Verification items for the finished model (mm, model axes). A direction names the side the tool comes from. Coordinates: 2 decimals unless noted, no trailing zeros. Order: outer loops, then holes, each group sorted by start corner. A loop starts at its lowest first (then second) coordinate and runs counter-clockwise, first axis right, second up. Notation, with made-up numbers: (-29.5, -37) -> (-7.5, -37) arc R15 ccw to (-7.5, -22) -> close; hole circle Ø6 at (19, 15). An arc over 180 degrees is marked (long way). Write item = value, one per line. Start each with the question number.
1. Thickness scan on line 1 along X through (y, z) = (31.75, 1.15); line 2 along X through (y, z) = (8.5, 1.55); line 3 along X through (y, z) = (-6, 0.5). Record the ranges inside material, lowest first. Write a range as from..to.
2. Cross-section at C-C on y = 31.75. Record the cut outline in (x, z), plus the area to 3 significant figures.
3. Cross-section at A-A on y = -24.95. Record the cut outline in (x, z), plus the area to 3 significant figures.
4. Set-up check for faces 1 (the flat face through (-5, 3.468, 1)), 2 (the flat face through (-4, 0, -1)), 3 (the cylindrical face through (-4.474, -28.776, 2.986)): record each of +Z, -Z, +X, -X, +Y, -Y from which the full face is reachable in a straight line by a thin tool's end or side.
5. Release check for a two-part mould opening along Y. For faces 4 (the flat face through (-5, -8.005, 1)), 5 (the cylindrical face through (14.73, 34.58, 3.4)), 6 (the cylindrical face through (-40.688, 0.464, 3.399)), 7 (the cylindrical face through (27.8, -25, 1.5)) record: +Y half, -Y half, draft (parallel to the pull), parting line (faces both ways), or undercut.
6. Cross-section at B-B on x = -19.5. Give the number of separate pieces and of enclosed holes in the cut face, plus the area to 3 significant figures.
7. Go/stop test with flat-tipped pins: P1, Ø1, axis at y = 16.5, z = 1.5, coming from the +X side; P2, Ø5, axis at x = -24, y = 19.5, coming from the -Z side; P3, Ø0.5, axis at y = 29.5, z = -0.5, coming from the +X side. Record where each tip stops, or that it passes through.
from build123d import *

# Parameters (mm, degrees)
SKETCH141_W          = 73.258
SKETCH141_H          = 70.3
SKETCH141_R          = 1.75
PAD050_DEPTH         = 4
FILLET012_R          = 2
SKETCH142_W          = 2
SKETCH142_H          = 70.3
POCKET059_DEPTH      = 2.1
SKETCH143_R          = 3
POCKET060_DEPTH      = 2.001
PAD051_DEPTH         = 1
POCKET061_DEPTH      = 1.001
POCKET061_DEPTH_BACK = 4.001


with BuildPart() as part:
    # Sketch141 → Pad050 (new body)
    with BuildSketch(Plane.XY):
        with Locations((-4.629, 0)):
            Rectangle(SKETCH141_W, SKETCH141_H)
        with Locations((-4.083, 31.75)):
            Circle(SKETCH141_R, mode=Mode.SUBTRACT)
        with Locations((-4.083, -31.75)):
            Circle(SKETCH141_R, mode=Mode.SUBTRACT)
    extrude(amount=PAD050_DEPTH)

    # Fillet012
    fillet012_edges = [part.edges().sort_by_distance(p)[0] for p in [
        (-4.629, 35.15, 4),
        (-41.258, 0, 4),
        (-41.258, 35.15, 2),
        (-41.258, -35.15, 2),
        (-4.629, -35.15, 4),
    ]]
    fillet(fillet012_edges, radius=FILLET012_R)

    # Sketch142 → Pocket059 (cut)
    with BuildSketch(Plane.XY):
        with Locations((31, 0)):
            Rectangle(SKETCH142_W, SKETCH142_H)
    extrude(amount=POCKET059_DEPTH, mode=Mode.SUBTRACT)

    # Sketch143 → Pocket060 (cut, through all)
    with BuildSketch(Plane.XY.offset(2)):
        with Locations((-4.083, 31.75)):
            Circle(SKETCH143_R)
        with Locations((-4.083, -31.75)):
            Circle(SKETCH143_R)
    extrude(amount=POCKET060_DEPTH, mode=Mode.SUBTRACT)

    # Sketch144 → Pad051 (join)
    with BuildSketch(Plane.XY):
        Polygon((-39.058, 32.95), (-9.108, 32.95), (-9.108, 28.15), (0.942, 28.15), (0.942, 32.95), (29.8, 32.95), (29.8, -32.95), (0.942, -32.95), (0.942, -28.15), (-9.108, -28.15), (-9.108, -32.95), (-39.058, -32.95), align=None)
    extrude(amount=-PAD051_DEPTH)

    # Sketch145 → Pocket061 (cut, two sides)
    with BuildSketch(Plane.XY) as pocket061_sk:
        with BuildLine():
            ThreePointArc((-35.858, 26.15), (-37.058, 24.95), (-35.858, 23.75))
            Line((-35.858, 23.75), (26.6, 23.75))
            ThreePointArc((26.6, 23.75), (27.8, 24.95), (26.6, 26.15))
            Line((-35.858, 26.15), (26.6, 26.15))
        make_face()
        with BuildLine():
            ThreePointArc((-35.858, 21.613636), (-37.058, 20.413636), (-35.858, 19.213636))
            Line((-35.858, 19.213636), (26.6, 19.213636))
            ThreePointArc((26.6, 19.213636), (27.8, 20.413636), (26.6, 21.613636))
            Line((-35.858, 21.613636), (26.6, 21.613636))
        make_face()
        with BuildLine():
            ThreePointArc((-35.858, 17.077273), (-37.058, 15.877273), (-35.858, 14.677273))
            Line((-35.858, 14.677273), (26.6, 14.677273))
            ThreePointArc((26.6, 14.677273), (27.8, 15.877273), (26.6, 17.077273))
            Line((-35.858, 17.077273), (26.6, 17.077273))
        make_face()
        with BuildLine():
            ThreePointArc((-35.858, 12.540909), (-37.058, 11.340909), (-35.858, 10.140909))
            Line((-35.858, 10.140909), (26.6, 10.140909))
            ThreePointArc((26.6, 10.140909), (27.8, 11.340909), (26.6, 12.540909))
            Line((-35.858, 12.540909), (26.6, 12.540909))
        make_face()
        with BuildLine():
            ThreePointArc((-35.858, 8.004545), (-37.058, 6.804545), (-35.858, 5.604545))
            Line((-35.858, 5.604545), (26.6, 5.604545))
            ThreePointArc((26.6, 5.604545), (27.8, 6.804545), (26.6, 8.004545))
            Line((-35.858, 8.004545), (26.6, 8.004545))
        make_face()
        with BuildLine():
            ThreePointArc((-35.858, 3.468182), (-37.058, 2.268182), (-35.858, 1.068182))
            Line((-35.858, 1.068182), (26.6, 1.068182))
            ThreePointArc((26.6, 1.068182), (27.8, 2.268182), (26.6, 3.468182))
            Line((-35.858, 3.468182), (26.6, 3.468182))
        make_face()
        with BuildLine():
            ThreePointArc((-35.858, -1.068182), (-37.058, -2.268182), (-35.858, -3.468182))
            Line((-35.858, -3.468182), (26.6, -3.468182))
            ThreePointArc((26.6, -3.468182), (27.8, -2.268182), (26.6, -1.068182))
            Line((-35.858, -1.068182), (26.6, -1.068182))
        make_face()
        with BuildLine():
            ThreePointArc((-35.858, -5.604545), (-37.058, -6.804545), (-35.858, -8.004545))
            Line((-35.858, -8.004545), (26.6, -8.004545))
            ThreePointArc((26.6, -8.004545), (27.8, -6.804545), (26.6, -5.604545))
            Line((-35.858, -5.604545), (26.6, -5.604545))
        make_face()
        with BuildLine():
            ThreePointArc((-35.858, -10.140909), (-37.058, -11.340909), (-35.858, -12.540909))
            Line((-35.858, -12.540909), (26.6, -12.540909))
            ThreePointArc((26.6, -12.540909), (27.8, -11.340909), (26.6, -10.140909))
            Line((-35.858, -10.140909), (26.6, -10.140909))
        make_face()
        with BuildLine():
            ThreePointArc((-35.858, -14.677273), (-37.058, -15.877273), (-35.858, -17.077273))
            Line((-35.858, -17.077273), (26.6, -17.077273))
            ThreePointArc((26.6, -17.077273), (27.8, -15.877273), (26.6, -14.677273))
            Line((-35.858, -14.677273), (26.6, -14.677273))
        make_face()
        with BuildLine():
            ThreePointArc((-35.858, -19.213636), (-37.058, -20.413636), (-35.858, -21.613636))
            Line((-35.858, -21.613636), (26.6, -21.613636))
            ThreePointArc((26.6, -21.613636), (27.8, -20.413636), (26.6, -19.213636))
            Line((-35.858, -19.213636), (26.6, -19.213636))
        make_face()
        with BuildLine():
            ThreePointArc((-35.858, -23.75), (-37.058, -24.95), (-35.858, -26.15))
            Line((-35.858, -26.15), (26.6, -26.15))
            ThreePointArc((26.6, -26.15), (27.8, -24.95), (26.6, -23.75))
            Line((-35.858, -23.75), (26.6, -23.75))
        make_face()
    extrude(amount=-POCKET061_DEPTH, mode=Mode.SUBTRACT)
    extrude(pocket061_sk.sketch, amount=POCKET061_DEPTH_BACK, mode=Mode.SUBTRACT)


solid = part.part
Worked out:
q1.line_1 = -41.26..-5.83, -2.33..30
q1.line_2 = -41.26..30
q1.line_3 = -41.26..-36.75, 27.49..30
q2.outline = (-41.26, 0) -> (-39.06, 0) -> (-39.06, -1) -> (-9.11, -1) -> (-9.11, 0) -> (-5.83, 0) -> (-5.83, 2) -> (-7.08, 2) -> (-7.08, 4) -> (-39.26, 4) arc R2 ccw to (-41.26, 2) -> close; (-2.33, 0) -> (0.94, 0) -> (0.94, -1) -> (29.8, -1) -> (29.8, 0) -> (30, 0) -> (30, 2.1) -> (32, 2.1) -> (32, 4) -> (-1.08, 4) -> (-1.08, 2) -> (-2.33, 2) -> close
q2.area = 328 mm²
q3.outline = (-41.26, 0) -> (-39.06, 0) -> (-39.06, -1) -> (-37.06, -1) -> (-37.06, 4) -> (-39.26, 4) arc R2 ccw to (-41.26, 2) -> close; (27.8, -1) -> (29.8, -1) -> (29.8, 0) -> (30, 0) -> (30, 2.1) -> (32, 2.1) -> (32, 4) -> (27.8, 4) -> close
q3.area = 32.5 mm²
q4.face_1 = +Z, -Z
q4.face_2 = -Z, +X, -X, +Y, -Y
q4.face_3 = +Z
q5.face_4 = undercut
q5.face_5 = +Y half
q5.face_6 = draft
q5.face_7 = undercut
q6.separate_pieces = 13
q6.enclosed_holes = 0
q6.area = 201 mm²
q7.P1 = 30
q7.P2 = -1
q7.P3 = 29.8
